```python
from build123d import *

# Parameters (mm, degrees)
BOSS_EXTRUDE1_DEPTH = 9
FILLET1_R           = 1


with BuildPart() as part:
    # Sketch1 → Boss-Extrude1 (new body)
    with BuildSketch(Plane(origin=(0, 0, 0), x_dir=(1, 0, 0), z_dir=(0, 1, 0))):
        with BuildLine():
            Line((-12, 20.652247549), (-12, 10.069242304))
            ThreePointArc((-12, 10.069242304), (0, 4.652247549), (12, 10.069242304))
            Line((12, 10.069242304), (12, 20.652247549))
            ThreePointArc((12, 20.652247549), (0, 32.652247549), (-12, 20.652247549))
        make_face()
    extrude(amount=BOSS_EXTRUDE1_DEPTH)

    # Fillet1
    fillet1_edges = [part.edges().sort_by_distance(p)[0] for p in [
        (12, 9, -15.360744926),
        (0, 9, -32.652247549),
        (12, 0, -15.360744926),
        (-12, 0, -15.360744926),
        (0, 0, -32.652247549),
        (-12, 9, -15.360744926),
    ]]
    fillet(fillet1_edges, radius=FILLET1_R)


solid = part.part
```
Design review of the part built by this model. Coordinates are the model's own, in mm. Coordinates: 2 decimals unless noted, no trailing zeros. Loops run counter-clockwise (first coordinate to the right, second up) from the corner with the lowest first, then second, coordinate; pieces in that order, holes last. Notation, with made-up numbers: M 46.5,23 L 71.5,23 A21 ccw 71.5,60 Z; hole C 69,18.25 d11. An arc over 180 degrees is marked long. One line per question, with ' | ' between items.
(1) We need section A-A (y = 4.5). Give the boundary of the cut face in (x, z).
Filled in:
outline: M -12,-20.65 A12 ccw 12,-20.65 L 12,-10.07 A16 ccw -12,-10.07 Z
(2) Wall thickness on probe 1 along Y at (x, z) = (-9.25, -28); probe 2 along Z at (x, y) = (0.75, 8.25); probe 3 along Z at (x, y) = (-4.5, 3.5): over which ranges is each line inside the solid? List them lowest first.
Filled in:
probe 1: y = 0.42 to 8.58 | probe 2: z = -32.6 to -4.67 | probe 3: z = -31.78 to -5.3
(3) For pin 1 Ø3 at (x, y) = (-3, 2) entering from -Z; pin 2 Ø1.5 at (x, y) = (4, 2.5) entering from -Z, all flat-tipped, find the tip position at first contact; note any pin that passes through.
Filled in:
pin 1: stops at z = -32.56 | pin 2: stops at z = -32.2
